Input: part model. Units: mm. Frame: model coordinates. Face numbers are marked on the shaded views. A direction names the side the tool comes from. Give positions to 0.01 mm unless a question says otherwise; leave off trailing zeros. Loops run counter-clockwise (first coordinate to the right, second up) from the corner with the lowest first, then second, coordinate; pieces in that order, holes last. Notation, with made-up numbers: (20, -20.5) - (64, -20.5) arc R25 ccw to (64, -4.5) - close; hole circle Ø11 at (61, 59). An arc over 180 degrees is marked (long way). One line per item, written item: value.
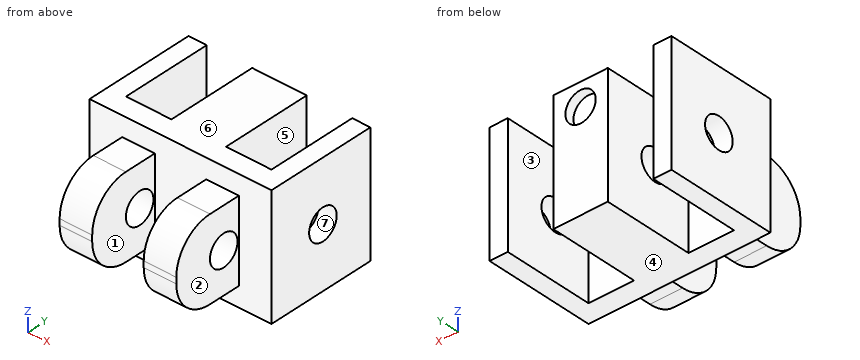
from build123d import *

# Parameters (mm, degrees)
BOSS_EXTRUDE1_DEPTH     = 54
CUT_EXTRUDE1_DEPTH      = 145.623649518
CUT_EXTRUDE1_DEPTH_BACK = 145.623649518
SKETCH2_R               = 10.25
CUT_EXTRUDE2_DEPTH      = 145.623649518
CUT_EXTRUDE2_DEPTH_BACK = 145.623649518
SKETCH3_R               = 10.25
CUT_EXTRUDE3_DEPTH      = 101.578327685
CUT_EXTRUDE3_DEPTH_BACK = 101.578327685
SKETCH4_W               = 21.5
SKETCH4_H               = 46.5
FILLET1_R               = 25
SKETCH5_W               = 120
SKETCH5_H               = 13
BOSS_EXTRUDE2_DEPTH     = 73.5
SKETCH6_W               = 30
SKETCH6_H               = 80
CUT_EXTRUDE4_DEPTH      = 60
SKETCH7_R               = 10
CUT_EXTRUDE5_DEPTH      = 6


with BuildPart() as part:
    # Sketch1 → Boss-Extrude1 (new body)
    with BuildSketch(Plane.XY):
        Polygon((60, 60), (-60, 60), (-60, -60), (-17, -60), (-17, -13.5), (17, -13.5), (17, -60), (60, -60), align=None)
    extrude(amount=BOSS_EXTRUDE1_DEPTH)

    # Sketch2 → Cut-Extrude1 (cut, two sides: drawn at the far end of the back side and taken through both)
    with BuildSketch(Plane(origin=(60, 0, 0), x_dir=(0, 0, -1), z_dir=(1, 0, 0)).offset(-CUT_EXTRUDE1_DEPTH_BACK)):
        with Locations(Location((-27, -24.75, 0), (0, 0, 90))):
            Circle(SKETCH2_R)
    extrude(amount=CUT_EXTRUDE1_DEPTH + CUT_EXTRUDE1_DEPTH_BACK, mode=Mode.SUBTRACT)

    # Sketch3 → Cut-Extrude2 (cut, two sides: drawn at the far end of the back side and taken through both)
    with BuildSketch(Plane(origin=(60, 0, 0), x_dir=(0, 0, -1), z_dir=(1, 0, 0)).offset(-CUT_EXTRUDE2_DEPTH_BACK)):
        with Locations(Location((-27, 24.75, 0), (0, 0, 90))):
            Circle(SKETCH3_R)
    extrude(amount=CUT_EXTRUDE2_DEPTH + CUT_EXTRUDE2_DEPTH_BACK, mode=Mode.SUBTRACT)

    # Sketch4 → Cut-Extrude3 (cut, two sides: drawn at the far end of the back side and taken through both)
    with BuildSketch(Plane.XY.offset(54).offset(-CUT_EXTRUDE3_DEPTH_BACK)):
        with Locations((-49.25, -36.75)):
            Rectangle(SKETCH4_W, SKETCH4_H)
        with Locations((49.25, -36.75)):
            Rectangle(SKETCH4_W, SKETCH4_H)
    extrude(amount=CUT_EXTRUDE3_DEPTH + CUT_EXTRUDE3_DEPTH_BACK, mode=Mode.SUBTRACT)

    # Fillet1
    fillet1_edges = [part.edges().sort_by_distance(p)[0] for p in [
        (27.75, -60, 0),
        (27.75, -60, 54),
        (-27.75, -60, 0),
        (-27.75, -60, 54),
    ]]
    fillet(fillet1_edges, radius=FILLET1_R)

    # Sketch5 → Boss-Extrude2 (add)
    with BuildSketch(Plane(origin=(0, 60, 0), x_dir=(1, 0, 0), z_dir=(0, 1, 0))):
        with Locations((0, 6.5)):
            Rectangle(SKETCH5_W, SKETCH5_H)
        with Locations((0, -60.5)):
            Rectangle(SKETCH5_W, SKETCH5_H)
    extrude(amount=-BOSS_EXTRUDE2_DEPTH)

    # Sketch6 → Cut-Extrude4 (cut)
    with BuildSketch(Plane(origin=(0, 60, 0), x_dir=(1, 0, 0), z_dir=(0, 1, 0))):
        with Locations((-33, -27)):
            Rectangle(SKETCH6_W, SKETCH6_H)
        with Locations((33, -27)):
            Rectangle(SKETCH6_W, SKETCH6_H)
    extrude(amount=-CUT_EXTRUDE4_DEPTH, mode=Mode.SUBTRACT)

    # Sketch7 → Cut-Extrude5 (cut)
    with BuildSketch(Plane(origin=(0, 60, 0), x_dir=(1, 0, 0), z_dir=(0, 1, 0))):
        with Locations(Location((0, -52, 0), (0, 0, 270))):
            Circle(SKETCH7_R)
    extrude(amount=-CUT_EXTRUDE5_DEPTH, mode=Mode.SUBTRACT)


solid = part.part
Item 1: Access query for the marked faces 1, 2 and 3. Directions: +Z, -Z, +X, -X, +Y, -Y. A direction counts if a zero-diameter tool reaches every point of the face in a straight line with its end or side. Return the directions, or none.
Verdict:
face 1: +Z, -Z, -Y
face 2: +Z, -Z, +X, -Y
face 3: +Z, -Z, +Y
Item 2: Pin query (flat end, axial travel): P1, Ø23.5, axis at y = -40.5, z = 31, coming from the -X side; P2, Ø1, axis at x = 22, z = 37.5, coming from the +Y side; P3, Ø17, axis at x = 27.5, y = -26.5, coming from the -Z side. Return the tip coordinate at first contact, or that it passes through.
Verdict:
P1: stops at x = -38.5
P2: stops at y = 0
P3: stops at z = 0
Item 3: Section C-C, the plane y = -24.75. Output: boundary loops of the cut face in (x, z), and give its area (3 significant figures).
Verdict:
outline: (-38.5, 0) - (-17, 0) - (-17, 16.75) - (-38.5, 16.75) - close; (-38.5, 37.25) - (-17, 37.25) - (-17, 54) - (-38.5, 54) - close; (17, 0) - (38.5, 0) - (38.5, 16.75) - (17, 16.75) - close; (17, 37.25) - (38.5, 37.25) - (38.5, 54) - (17, 54) - close
area: 1,440 mm^2
Item 4: Material intervals for L1, parallel to X at y = 13, z = -5; L2, parallel to X at y = 57.4, z = 52; L3, parallel to Y at x = 50.5, z = 26.5, sorted ascending.
Verdict:
L1: x = -60 to -48, -18 to 18, 48 to 60
L2: x = -60 to -48, -18 to -10, 10 to 18, 48 to 60
L3: y = -13.5 to 14.51, 34.99 to 60
Item 5: Section B-B, the plane x = 20. Output: boundary loops of the cut face in (y, z).
Verdict:
outline: (-60, 25) arc R25 ccw to (-35, 0) - (-13.5, 0) - (-13.5, -13) - (0, -13) - (0, 67) - (-13.5, 67) - (-13.5, 54) - (-35, 54) arc R25 ccw to (-60, 29) - close; hole circle Ø20.5 at (-24.75, 27)
Item 6: Draft query along Z for the marked faces 4, 5, 6 and 7. Return one class per face: pulls with the +Z half, pulls with the -Z half, needs draft (parallel to the pull), parting line crosses it, or undercut.
Verdict:
face 4: pulls with the -Z half
face 5: needs draft
face 6: pulls with the +Z half
face 7: undercut
Item 7: Section D-D, the plane z = 27. Count the separate pieces of the cut face and the enclosed holes in it, and give its area (3 significant figures).
Verdict:
separate pieces: 6
enclosed holes: 0
area: 5,110 mm^2
Item 8: Section A-A, the plane y = 48.5. Output: boundary loops of the cut face in (x, z).
Verdict:
outline: (-60, -13) - (-48, -13) - (-48, 67) - (-60, 67) - close; (-18, -13) - (18, -13) - (18, 67) - (-18, 67) - close; (48, -13) - (60, -13) - (60, 67) - (48, 67) - close
